Input: part model. Units: mm. Frame: model coordinates. A direction names the side the tool comes from. Coordinates: 2 decimals unless noted, no trailing zeros. Order: outer loops, then holes, each group sorted by start corner. A loop starts at its lowest first (then second) coordinate and runs counter-clockwise, first axis right, second up. Notation, with made-up numbers: (79, 83) - (124, 83) arc R18 ccw to (124, 108) - close; hole circle Ø5 at (13, 3). An arc over 180 degrees is marked (long way). Answer as CSV lines item,"result". Start each with the question number.
Item 1: Section B-B (x = 7.5). Output: boundary loops of the cut face in (y, z).
Item 2: First-contact query: pin 1 (6.5 mm diameter, centred on x = -8, y = 4.5, fed in from -Z); pin 2 (2.5 mm diameter, centred on x = -102, y = -1.5, fed in from +Z); pin 3 (4 mm diameter, centred on x = -5.5, y = 1.5, fed in from +Z). Flat tips, straight axial feed; report the tip coordinate or a pass-through.
Item 3: Draft query along X for faces 4 (the flat face through (17.64, -1.3, 9.86)), 5 (the cylindrical face through (39.967, -2.465, 11.617)), 6 (the flat face through (22.589, 4.257, 9.86)). Return one class per face: +X half, -X half, draft (parallel to the pull), parting line (faces both ways), or undercut.
Item 4: Section A-A (z = 10). Output: boundary loops of the cut face in (x, y), and give its area (3 significant figures).
Item 5: Section D-D (z = 24). Output: boundary loops of the cut face in (x, y), and give its area (3 significant figures).
Item 6: Material intervals for line 1 along Z through (x, y) = (-103, -1.25); line 2 along Y through (x, z) = (-15, 38.5); line 3 along X through (y, z) = (-0.5, 34.5), sorted ascending.
Item 7: Section C-C (y = -3.25). Output: boundary loops of the cut face in (x, z), and give its area (3 significant figures).
Item 8: Access query for faces 1 (the flat face through (-38, -5, 10)), 2 (the flat face through (-85, -2, 0)), 3 (the flat face through (-85, -2, 20)). Directions: +Z, -Z, +X, -X, +Y, -Y. A direction counts if a zero-diameter tool reaches every point of the face in a straight line with its end or side. Return the directions, or none.
Autodesk Inventor part; units mm, degrees
ref_plane "YZ Plane" through (0, 0, 0) normal (1, 0, 0) x (0, 1, 0)
ref_plane "XZ Plane" through (0, 0, 0) normal (0, 1, 0) x (-1, 0, 0)
ref_plane "XY Plane" through (0, 0, 0) normal (0, 0, 1) x (1, 0, 0)
sketch "Sketch1" plane through (0, 0, 0) normal (0, 0, 1) x (1, 0, 0)
  line L0 (0, 0) -> (-50, 0)
  line L1 (-50, 0) -> (-50, -5)
  line L2 (-50, -5) -> (0, -5)
  line L3 (0, -5) -> (0, 0)
  line L4 (0, 0) -> (19.6962, 3.473)
  line L5 (0, 0) -> (20, 0) construction
  line L6 (19.6962, 3.473) -> (18.8279, 8.397)
  line L7 (18.8279, 8.397) -> (-28.7939, 0)
  line L8 (0, 0) -> (-28.3564, -5)
  line L9 (0, 0) -> (28.7939, 0) construction
  line L10 (-50, 0) -> (-130, 0)
  line L11 (-130, 0) -> (-130, -5)
  line L12 (-130, -5) -> (-50, -5)
  line L13 (18.8279, 8.397) -> (31, -5)
  line L14 (31, -5) -> (21, -5)
  line L15 (21, -5) -> (10.5825, 6.4659)
  line L16 (31, -5) -> (31, 0)
  line L17 (31, 0) -> (26.4572, 0)
  line L18 (31, 0) -> (36, 0)
  line L19 (36, 0) -> (36, -5)
  line L20 (36, -5) -> (31, -5)
  line L21 (31, -5) -> (31, 0)
  point P0 (14.1847, 2.5011)
  point P1 (31, -5)
  dimension "d0" = 50
  dimension "d1" = 5
  dimension "d2" = 20
  dimension "d3" = 10
  dimension "d4" = 5
  dimension "d5" = 90
  dimension "d11" = 170
  dimension "d12" = 80
  dimension "d16" = 5
extrude "Extrusion1" add sketch "Sketch1" along normal blind 20 contours L8 L2 L1 L0 | L0 L7 L6 L4 | L4 L6 L13 L14 L15 | L1 L12 L11 L10 | L17 L16 L13 | L16 L18 L19 L20
sketch "Sketch2" plane through (-28.7939, 0, 0) normal (-0.1736, 0.9848, 0) x (-0.9848, -0.1736, 0)
  line L0 (-48.3564, 0) -> (0, 0)
  line L1 (0, 0) -> (0, 20)
  line L2 (-48.3564, 20) -> (0, 20)
  line L3 (-48.3564, 0) -> (-48.3564, 20)
  line L4 (-48.3564, 10) -> (0, 10)
  line L5 (-24.1782, 20) -> (-24.1782, 0)
  line L6 (-28.3564, 0) -> (-48.3564, 0)
  circle A0 centre (-24.1782, 10) radius 2.75
  dimension "d8" = 5.5
extrude "Extrusion2" cut sketch "Sketch2" against normal blind 20 contours A0 L5 L4 | L4 L5 A0 | L5 L4 A0 | L5 A0 L4
sketch "Sketch3" plane through (0, 0, 0) normal (0, 1, 0) x (-1, 0, 0)
  line L0 (130, 0) -> (28.3564, 0)
  line L1 (28.3564, 0) -> (28.3564, 20)
  line L2 (130, 20) -> (28.3564, 20)
  line L3 (130, 0) -> (130, 20)
  line L4 (-18.8279, 0) -> (28.7939, 0)
  line L5 (28.3564, 20) -> (28.7939, 0)
  line L6 (28.3564, 0) -> (28.3564, 20)
  line L7 (28.3564, 10) -> (-19.6962, 10)
  line L8 (-19.6962, 0) -> (-19.6962, 20)
  line L9 (28.7939, 0) -> (130, 0)
  circle A0 centre (0, 10) radius 30.4809
  circle A1 centre (0, 10) radius 40
  point P0 (0, 0)
  point P1 (38.7298, 20)
  point P2 (38.7298, 0)
  point P3 (28.7939, 20)
  dimension "d13" = 80
extrude "Extrusion3" add sketch "Sketch3" against normal blind 5 contours L0 A1 L2 A0 picked at (-11.3499, -24.8055)
properties part number "base mount for central centrifuge"
Determined:
1,outline,"(-5, -29.29) - (0, -29.29) - (0, -19.54) - (-5, -19.54) - close; (-5, 39.54) - (0, 39.54) - (0, 49.29) - (-5, 49.29) - close; (1.32, 0) - (6.4, 0) - (6.4, 20) - (1.32, 20) - close"
2,pin 1,"stops at z = 0"
2,pin 2,"stops at z = 20"
2,pin 3,"stops at z = 49.78"
3,face 4,"undercut"
3,face 5,"parting line"
3,face 6,"+X half"
4,outline,"(-130, -5) - (-28.36, -5) - (-6.82, -1.2) - (-7.69, 3.72) - (-28.79, 0) - (-130, 0) - close; (-2.27, 4.68) - (-1.41, -0.25) - (0, 0) - (14.18, 2.5) - (21, -5) - (40, -5) - (40, 0) - (26.46, 0) - (18.83, 8.4) - close"
4,area,"869 mm^2"
5,outline,"(-37.47, -5) - (-27.08, -5) - (-27.08, 0) - (-37.47, 0) - close; (27.08, -5) - (37.47, -5) - (37.47, 0) - (27.08, 0) - close"
5,area,"104 mm^2"
6,line 1,"z = 0 to 20"
6,line 2,"y = -5 to 0"
6,line 3,"x = -31.62 to -18.13, 18.13 to 31.62"
7,outline,"(-130, 0) - (-38.73, 0) arc R40 ccw (long way) to (-38.73, 20) - (-130, 20) - close; hole (-28.79, 0) arc R30.48 ccw to (28.79, 0) - (19.41, 0) - (19.41, 20) - (28.79, 20) arc R30.48 ccw to (-28.79, 20) - (-18.43, 20) - (-18.43, 0) - close"
7,area,"4,360 mm^2"
8,face 1,"+Z, -Z, +X, -X, -Y"
8,face 2,"-Z, -X, +Y, -Y"
8,face 3,"+Z, -X, +Y, -Y"
